```python
from build123d import *

# Parameters (mm, degrees)
SKETCH2_R           = 2.5
SKETCH2_R_2         = 4.5
SKETCH2_R_3         = 8
SKETCH2_R_4         = 2
BOSS_EXTRUDE1_DEPTH = 6.7


with BuildPart() as part:
    # Sketch2 → Boss-Extrude1 (new body)
    with BuildSketch(Plane(origin=(0, 0, 0), x_dir=(1, 0, 0), z_dir=(0, 1, 0))):
        Polygon((275.201010127, -365), (295, -345.201010127), (295, 306.310137162), (236.310137162, 365), (-236.310137162, 365), (-295, 306.310137162), (-295, -345.201010127), (-275.201010127, -365), align=None)
        with Locations(Location((-265, -326, 0), (0, 0, 270))):
            Circle(SKETCH2_R, mode=Mode.SUBTRACT)
        with Locations(Location((-265, -306, 0), (0, 0, 270))):
            Circle(SKETCH2_R, mode=Mode.SUBTRACT)
        with Locations(Location((-199, -240.38125, 0), (0, 0, 270))):
            Circle(SKETCH2_R_2, mode=Mode.SUBTRACT)
        with Locations(Location((-125, -343, 0), (0, 0, 270))):
            Circle(SKETCH2_R_2, mode=Mode.SUBTRACT)
        with Locations(Location((-40, -343, 0), (0, 0, 270))):
            Circle(SKETCH2_R, mode=Mode.SUBTRACT)
        with Locations(Location((-40, -263, 0), (0, 0, 270))):
            Circle(SKETCH2_R, mode=Mode.SUBTRACT)
        with Locations(Location((-40, -183, 0), (0, 0, 270))):
            Circle(SKETCH2_R, mode=Mode.SUBTRACT)
        with Locations(Location((-265, -80, 0), (0, 0, 270))):
            Circle(SKETCH2_R, mode=Mode.SUBTRACT)
        with Locations(Location((-265, -60, 0), (0, 0, 270))):
            Circle(SKETCH2_R, mode=Mode.SUBTRACT)
        with Locations(Location((-180, -16, 0), (0, 0, 270))):
            Circle(SKETCH2_R, mode=Mode.SUBTRACT)
        with Locations(Location((40, -343, 0), (0, 0, 270))):
            Circle(SKETCH2_R, mode=Mode.SUBTRACT)
        with Locations(Location((125, -343, 0), (0, 0, 270))):
            Circle(SKETCH2_R_2, mode=Mode.SUBTRACT)
        with Locations(Location((40, -263, 0), (0, 0, 270))):
            Circle(SKETCH2_R, mode=Mode.SUBTRACT)
        with Locations(Location((40, -183, 0), (0, 0, 270))):
            Circle(SKETCH2_R, mode=Mode.SUBTRACT)
        with Locations(Location((265, -326, 0), (0, 0, 270))):
            Circle(SKETCH2_R, mode=Mode.SUBTRACT)
        with Locations(Location((265, -306, 0), (0, 0, 270))):
            Circle(SKETCH2_R, mode=Mode.SUBTRACT)
        with Locations(Location((199, -240.38125, 0), (0, 0, 270))):
            Circle(SKETCH2_R_2, mode=Mode.SUBTRACT)
        with Locations(Location((0, -16, 0), (0, 0, 270))):
            Circle(SKETCH2_R, mode=Mode.SUBTRACT)
        with Locations(Location((180, -16, 0), (0, 0, 270))):
            Circle(SKETCH2_R, mode=Mode.SUBTRACT)
        with Locations(Location((265, -80, 0), (0, 0, 270))):
            Circle(SKETCH2_R, mode=Mode.SUBTRACT)
        with Locations(Location((265, -60, 0), (0, 0, 270))):
            Circle(SKETCH2_R, mode=Mode.SUBTRACT)
        with Locations(Location((-227.53125, 15, 0), (0, 0, 270))):
            Circle(SKETCH2_R, mode=Mode.SUBTRACT)
        with Locations(Location((-227.53125, 45, 0), (0, 0, 270))):
            Circle(SKETCH2_R, mode=Mode.SUBTRACT)
        with Locations(Location((-199, 80, 0), (0, 0, 270))):
            Circle(SKETCH2_R_2, mode=Mode.SUBTRACT)
        with Locations(Location((-180, 76, 0), (0, 0, 270))):
            Circle(SKETCH2_R, mode=Mode.SUBTRACT)
        with Locations(Location((-265, 166, 0), (0, 0, 270))):
            Circle(SKETCH2_R, mode=Mode.SUBTRACT)
        with Locations(Location((-125, 180.703125, 0), (0, 0, 270))):
            Circle(SKETCH2_R_2, mode=Mode.SUBTRACT)
        with Locations(Location((-40, 101, 0), (0, 0, 270))):
            Circle(SKETCH2_R, mode=Mode.SUBTRACT)
        with Locations(Location((-40, 181, 0), (0, 0, 270))):
            Circle(SKETCH2_R, mode=Mode.SUBTRACT)
        with Locations(Location((-265, 186, 0), (0, 0, 270))):
            Circle(SKETCH2_R, mode=Mode.SUBTRACT)
        Polygon((-275, 269.741594667), (-275, 298.025865914), (-228.025865914, 345), (-199.741594667, 345), align=None, mode=Mode.SUBTRACT)
        Polygon((-143.173052172, 345), (-275, 213.173052172), (-275, 241.457323419), (-171.457323419, 345), align=None, mode=Mode.SUBTRACT)
        with Locations(Location((-40, 261, 0), (0, 0, 270))):
            Circle(SKETCH2_R, mode=Mode.SUBTRACT)
        with Locations(Location((-30, 303.734375, 0), (0, 0, 270))):
            Circle(SKETCH2_R_3, mode=Mode.SUBTRACT)
        with Locations(Location((-40, 341, 0), (0, 0, 270))):
            Circle(SKETCH2_R, mode=Mode.SUBTRACT)
        with Locations(Location((-27.5, 333.5, 0), (0, 0, 270))):
            Circle(SKETCH2_R_4, mode=Mode.SUBTRACT)
        with Locations(Location((-27.5, 346, 0), (0, 0, 270))):
            Circle(SKETCH2_R_4, mode=Mode.SUBTRACT)
        with BuildLine():
            Line((172.2875, -10), (-172.2875, -10))
            ThreePointArc((-172.2875, -10), (-179.358567812, -7.071067812), (-182.2875, 0))
            Line((-182.2875, 0), (-182.2875, 60))
            ThreePointArc((-182.2875, 60), (-179.358567812, 67.071067812), (-172.2875, 70))
            Line((-172.2875, 70), (172.2875, 70))
            ThreePointArc((172.2875, 70), (179.358567812, 67.071067812), (182.2875, 60))
            Line((182.2875, 60), (182.2875, 0))
            ThreePointArc((182.2875, 0), (179.358567812, -7.071067812), (172.2875, -10))
        make_face(mode=Mode.SUBTRACT)
        with Locations(Location((0, 76, 0), (0, 0, 270))):
            Circle(SKETCH2_R, mode=Mode.SUBTRACT)
        with Locations(Location((40, 101, 0), (0, 0, 270))):
            Circle(SKETCH2_R, mode=Mode.SUBTRACT)
        with Locations(Location((40, 181, 0), (0, 0, 270))):
            Circle(SKETCH2_R, mode=Mode.SUBTRACT)
        with Locations(Location((125, 180.703125, 0), (0, 0, 270))):
            Circle(SKETCH2_R_2, mode=Mode.SUBTRACT)
        with Locations(Location((180, 76, 0), (0, 0, 270))):
            Circle(SKETCH2_R, mode=Mode.SUBTRACT)
        with Locations(Location((199, 80, 0), (0, 0, 270))):
            Circle(SKETCH2_R_2, mode=Mode.SUBTRACT)
        with Locations(Location((227.53125, 15, 0), (0, 0, 270))):
            Circle(SKETCH2_R, mode=Mode.SUBTRACT)
        with Locations(Location((227.53125, 45, 0), (0, 0, 270))):
            Circle(SKETCH2_R, mode=Mode.SUBTRACT)
        with Locations(Location((265, 166, 0), (0, 0, 270))):
            Circle(SKETCH2_R, mode=Mode.SUBTRACT)
        with Locations(Location((40, 261, 0), (0, 0, 270))):
            Circle(SKETCH2_R, mode=Mode.SUBTRACT)
        with Locations(Location((30, 303.734375, 0), (0, 0, 270))):
            Circle(SKETCH2_R_3, mode=Mode.SUBTRACT)
        with Locations(Location((27.5, 333.5, 0), (0, 0, 270))):
            Circle(SKETCH2_R_4, mode=Mode.SUBTRACT)
        with Locations(Location((27.5, 346, 0), (0, 0, 270))):
            Circle(SKETCH2_R_4, mode=Mode.SUBTRACT)
        with Locations(Location((40, 341, 0), (0, 0, 270))):
            Circle(SKETCH2_R, mode=Mode.SUBTRACT)
        with Locations(Location((265, 186, 0), (0, 0, 270))):
            Circle(SKETCH2_R, mode=Mode.SUBTRACT)
        Polygon((143.173052172, 345), (171.457323419, 345), (275, 241.457323419), (275, 213.173052172), align=None, mode=Mode.SUBTRACT)
        Polygon((199.741594667, 345), (228.025865914, 345), (275, 298.025865914), (275, 269.741594667), align=None, mode=Mode.SUBTRACT)
    extrude(amount=BOSS_EXTRUDE1_DEPTH)


solid = part.part
```
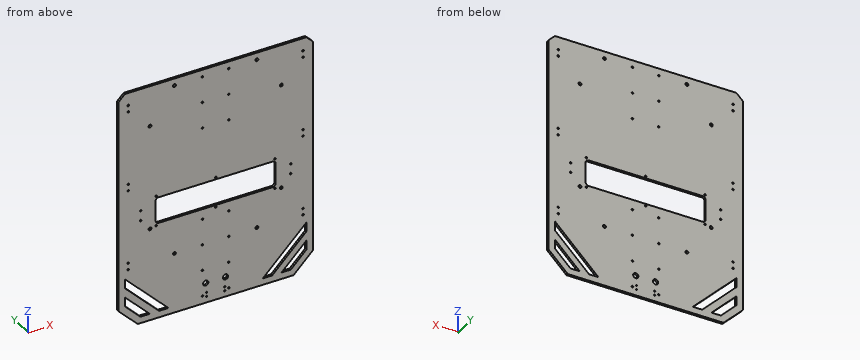
For this review, take the finished solid that the model builds, in its own axes (mm). Round coordinates to 2 decimals unless told otherwise and drop trailing zeros. Write each loop counter-clockwise with the first axis right and the second up, starting at its lowest first coordinate (ties: lowest second). Pieces come first, ordered by that corner, then holes. Notation, with made-up numbers: (-3, 22) -> (12, 22) arc R22 ccw to (12, 47) -> close; hole circle Ø2 at (31, -16). An arc over 180 degrees is marked (long way). Use one line per item in the form item = value.
1) Take a section at B-B, the plane z = -223. Write out the cut boundary in (x, y).
Found:
outline = (-295, 0) -> (-275, 0) -> (-275, 6.7) -> (-295, 6.7) -> close; (-265.17, 0) -> (265.17, 0) -> (265.17, 6.7) -> (-265.17, 6.7) -> close; (275, 0) -> (295, 0) -> (295, 6.7) -> (275, 6.7) -> close
2) Take a section at C-C, the plane y = 4. Count the separate pieces of the cut face and the enclosed holes in it, and give its area (3 significant figures).
Found:
separate_pieces = 1
enclosed_holes = 55
area = 386,000 mm2
3) Clearance check with a flat-ended pin moving along its axis: pin 1 (3 mm diameter, centred on x = 40, z = -181, fed in from -Y). State where the tip first meets the part, or that it passes through.
Found:
pin_1 = through
4) To check wall thickness, follow L1, parallel to X at y = 3.5, z = -14.5; L2, parallel to X at y = 3, z = 60; L3, parallel to X at y = 2.75, z = -15. State the ranges of each line that lie inside material, in increasing order. Write a range as from..to.
Found:
L1 = -295..-229.98, -225.08..-182.29, 182.29..225.08, 229.98..295
L2 = -295..-267.5, -262.5..262.5, 267.5..295
L3 = -295..-230.03, -225.03..-182.29, 182.29..225.03, 230.03..295
5) Take a section at A-A, the plane x = -105. Write out the cut boundary in (y, z).
Found:
outline = (0, -365) -> (6.7, -365) -> (6.7, -70) -> (0, -70) -> close; (0, 10) -> (6.7, 10) -> (6.7, 365) -> (0, 365) -> close
